For this review, use the dimensioned drawing (mm, ordinates from the lowest corner) and the shaded views. Round coordinates to 2 decimals unless told otherwise and drop trailing zeros. Write each loop counter-clockwise with the first axis right and the second up, starting at its lowest first coordinate (ties: lowest second). Pieces come first, ordered by that corner, then holes. Notation, with made-up numbers: (14.25, 61) -> (18.25, 61) arc R27 ccw to (18.25, 100) -> close; hole circle Ø4 at (-1, -23). An arc over 180 degrees is marked (long way). Answer as CSV lines item,"result". Start each with the question number.
Item 1: Take a section at B-B on x = 32.5. Give the boundary of the cut face in (y, z) (3 decimals), then the cut area to 3 significant figures.
Item 2: Wall thickness on probe 1 along Y at (x, z) = (32, 35) (3 decimals); probe 2 along Y at (x, z) = (51, 170) (3 decimals); probe 3 along X at (y, z) = (5, 71): over which ranges is each line inside the solid? List them lowest first. Write a range as from..to.
Item 3: For pin 1 Ø5.5 at (x, y) = (31.5, 26) entering from -Z, flat-tipped, find the tip position at first contact; note if it passes through.
Item 4: Take a section at C-C on y = 29. Give the boundary of the cut face in (x, z), then the cut area to 3 significant figures.
Item 5: Take a section at A-A on z = 25. Give the boundary of the cut face in (x, y), then the cut area to 3 significant figures.
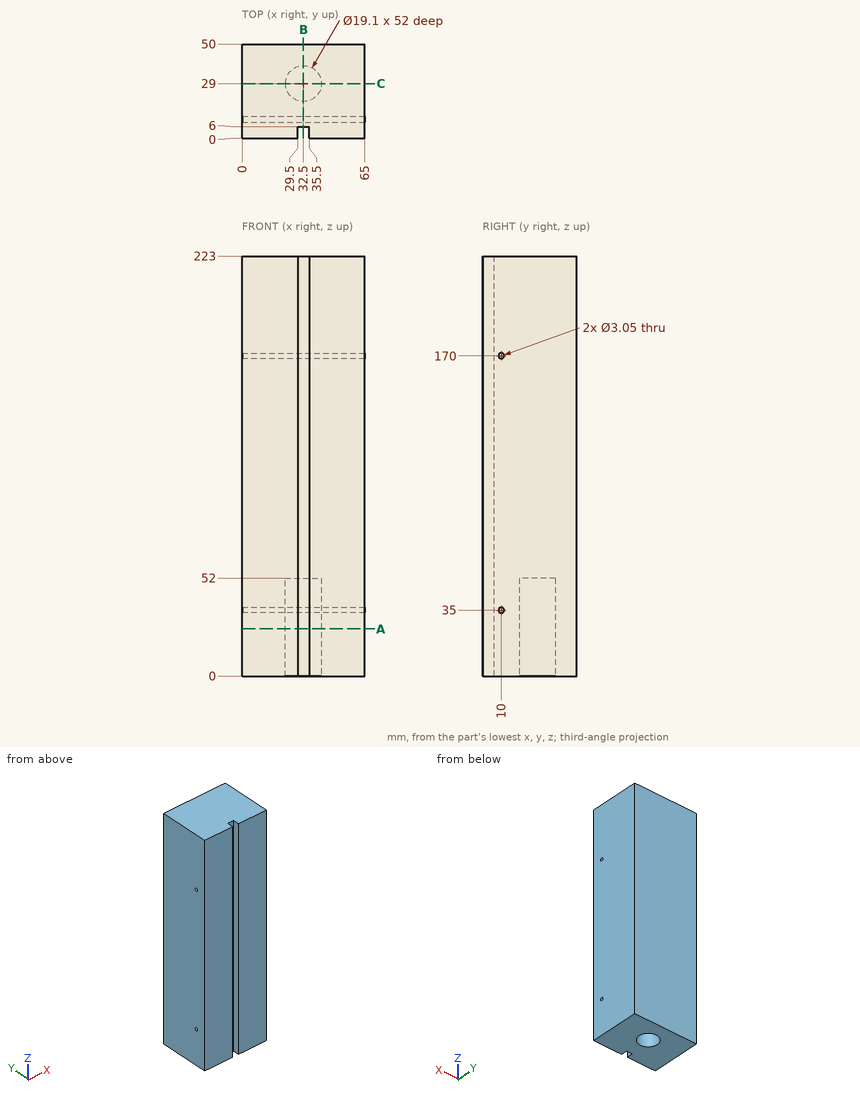
Output values:
1,outline,"(6, 0) -> (19.45, 0) -> (19.45, 52) -> (38.55, 52) -> (38.55, 0) -> (50, 0) -> (50, 223) -> (6, 223) -> close; hole circle Ø3.05 at (10, 35); hole circle Ø3.05 at (10, 170)"
1,area,"8,800 mm^2"
2,probe 1,"y = 6..8.475, 11.525..19.463, 38.537..50"
2,probe 2,"y = 0..8.475, 11.525..50"
2,probe 3,"x = 0..29.5, 35.5..65"
3,pin 1,"stops at z = 52"
4,outline,"(0, 0) -> (22.95, 0) -> (22.95, 52) -> (42.05, 52) -> (42.05, 0) -> (65, 0) -> (65, 223) -> (0, 223) -> close"
4,area,"13,500 mm^2"
5,outline,"(0, 0) -> (29.5, 0) -> (29.5, 6) -> (35.5, 6) -> (35.5, 0) -> (65, 0) -> (65, 50) -> (0, 50) -> close; hole circle Ø19.1 at (32.5, 29)"
5,area,"2,930 mm^2"
